```python
from build123d import *

# Parameters (mm, degrees)
F3_DEPTH = 24.4
F4_DEPTH = 2.4
F5_DEPTH = 13.4
F6_R     = 2


with BuildPart() as f3:
    # F2 (on Top) → F3 (new body)
    with BuildSketch(Plane.XY):
        with BuildLine():
            Line((-15.865, -9.0505248467), (-15.865, 0))
            Line((-15.865, 0), (-15.865, 9.0505248467))
            ThreePointArc((-15.865, 9.0505248467), (-17.6548074189, 4.68166637), (-18.265, 0))
            ThreePointArc((-18.265, 0), (-17.6548074189, -4.68166637), (-15.865, -9.0505248467))
        make_face()
        with BuildLine():
            ThreePointArc((-18.265, 0), (-17.6548074189, 4.68166637), (-15.865, 9.0505248467))
            Line((-15.865, 9.0505248467), (-15.865, 18.265))
            Line((-15.865, 18.265), (-18.265, 18.265))
            Line((-18.265, 18.265), (-18.265, 0))
        make_face()
        with BuildLine():
            Line((-15.865, -18.265), (-15.865, -9.0505248467))
            ThreePointArc((-15.865, -9.0505248467), (-17.6548074189, -4.68166637), (-18.265, 0))
            Line((-18.265, 0), (-18.265, -18.265))
            Line((-18.265, -18.265), (-15.865, -18.265))
        make_face()
        with BuildLine():
            Line((-15.865, 9.0505248467), (-15.865, 0))
            Line((-15.865, 0), (-15.865, -9.0505248467))
            ThreePointArc((-15.865, -9.0505248467), (4.68166637, -17.6548074189), (18.265, 0))
            ThreePointArc((18.265, 0), (4.68166637, 17.6548074189), (-15.865, 9.0505248467))
        make_face()
        with BuildLine():
            ThreePointArc((-15.865, 0), (0, 15.865), (15.865, 0))
            ThreePointArc((15.865, 0), (0, -15.865), (-15.865, 0))
        make_face(mode=Mode.SUBTRACT)
    extrude(amount=F3_DEPTH)

    # F2 (on Top) → F4 (join)
    with BuildSketch(Plane.XY):
        with BuildLine():
            Line((-15.865, 9.0505248467), (-15.865, 0))
            Line((-15.865, 0), (-15.865, -9.0505248467))
            ThreePointArc((-15.865, -9.0505248467), (4.68166637, -17.6548074189), (18.265, 0))
            ThreePointArc((18.265, 0), (4.68166637, 17.6548074189), (-15.865, 9.0505248467))
        make_face()
        with BuildLine():
            ThreePointArc((-15.865, 0), (0, 15.865), (15.865, 0))
            ThreePointArc((15.865, 0), (0, -15.865), (-15.865, 0))
        make_face(mode=Mode.SUBTRACT)
        with BuildLine():
            ThreePointArc((-15.865, 0), (0, -15.865), (15.865, 0))
            ThreePointArc((15.865, 0), (0, 15.865), (-15.865, 0))
        make_face()
        Polygon((-7.6111814104, 9.7325870595), (4.6230769329, 11.457769984), (12.2342583433, 1.7251829245), (7.6111814104, -9.7325870595), (-4.6230769329, -11.457769984), (-12.2342583433, -1.7251829245), align=None, mode=Mode.SUBTRACT)
        Polygon((12.2342583433, 1.7251829245), (4.6230769329, 11.457769984), (-7.6111814104, 9.7325870595), (-12.2342583433, -1.7251829245), (-4.6230769329, -11.457769984), (7.6111814104, -9.7325870595), align=None)
    extrude(amount=F4_DEPTH)

    # F2 (on Top) → F5 (join)
    with BuildSketch(Plane.XY):
        with BuildLine():
            ThreePointArc((-15.865, 0), (0, -15.865), (15.865, 0))
            ThreePointArc((15.865, 0), (0, 15.865), (-15.865, 0))
        make_face()
        Polygon((-7.6111814104, 9.7325870595), (4.6230769329, 11.457769984), (12.2342583433, 1.7251829245), (7.6111814104, -9.7325870595), (-4.6230769329, -11.457769984), (-12.2342583433, -1.7251829245), align=None, mode=Mode.SUBTRACT)
    extrude(amount=F5_DEPTH)

    # F6
    f6_edges = [f3.edges().sort_by_distance(p)[0] for p in [
        (-15.865, -9.050525, 12.2),
        (-15.865, 9.050525, 12.2),
    ]]
    fillet(f6_edges, radius=F6_R)


solid = f3.part
```
Input: part model. Units: mm. Frame: model coordinates. A direction names the side the tool comes from. Round coordinates to 2 decimals unless told otherwise and drop trailing zeros. Write each loop counter-clockwise with the first axis right and the second up, starting at its lowest first coordinate (ties: lowest second). Pieces come first, ordered by that corner, then holes. Notation, with made-up numbers: M 47,24 L 105,24 A20 ccw 105,48 Z; hole C 53,41 d3. An arc over 180 degrees is marked long. Write each question's results on one line, items separated by ' | '.
Q1. Section query B-B (x = 8.5). Return loops of the section in (y, z), and give its area (3 significant figures).
Results:
outline: M -16.17,0 L 16.17,0 L 16.17,24.4 L 13.4,24.4 L 13.4,13.4 L 6.5,13.4 L 6.5,2.4 L -7.53,2.4 L -7.53,13.4 L -13.4,13.4 L -13.4,24.4 L -16.17,24.4 Z | area: 340 mm^2
Q2. Section query D-D (z = 20). Return loops of the section in (x, y) (3 decimals).
Results:
outline: M -18.265,-18.265 L -15.865,-18.265 L -15.865,-14.779 A2 cw -12.497,-13.321 A18.265 ccw long -12.497,13.321 A2 cw -15.865,14.779 L -15.865,18.265 L -18.265,18.265 Z; hole C 0,0 d31.73
Q3. Pin query (flat end, axial travel): P1, Ø5, axis at x = 5.5, y = -11.5, coming from the -Z side; P2, Ø1.5, axis at x = -1, z = 18, coming from the -Y side; P3, Ø5, axis at y = 6, z = 17.5, coming from the +X side; P4, Ø3, axis at y = -4, z = 7, coming from the +X side. Return the tip coordinate at first contact, or that it passes through.
Results:
P1: stops at z = 0 | P2: stops at y = -18.26 | P3: stops at x = 17.93 | P4: stops at x = 18.09
Q4. Section query A-A (z = 7). Return loops of the section in (x, y) (3 decimals), and give its area (3 significant figures).
Results:
outline: M -18.265,-18.265 L -15.865,-18.265 L -15.865,-14.779 A2 cw -12.497,-13.321 A18.265 ccw long -12.497,13.321 A2 cw -15.865,14.779 L -15.865,18.265 L -18.265,18.265 Z; hole M -12.234,-1.725 L -4.623,-11.458 L 7.611,-9.733 L 12.234,1.725 L 4.623,11.458 L -7.611,9.733 Z | area: 721 mm^2
Q5. Draft query along X for faces 1 (the face through (8.375, 6.66, 7.823)), 2 (the face through (-17, 18.265, 12)), 3 (the face through (-18.265, 0, 12)). Return one class per face: released by +X, released by -X, zero draft, split by the parting line, or undercut.
Results:
face 1: undercut | face 2: zero draft | face 3: released by -X
Q6. Section query C-C (y = 6.5). Return loops of the section in (x, z) (1 decimal), and give its area (3 significant figures).
Results:
outline: M -18.3,0 L 17.1,0 L 17.1,24.4 L 14.5,24.4 L 14.5,13.4 L 8.5,13.4 L 8.5,2.4 L -8.9,2.4 L -8.9,13.4 L -14.5,13.4 L -14.5,24.4 L -18.3,24.4 Z | area: 352 mm^2
Q7. Access query for faces 4 (the face through (0, 0, 0)), 5 (the face through (-15.865, 16, 12)), 6 (the face through (-1.58, 10.583, 7.823)), 7 (the face through (-15.865, -17, 12)). Directions: +Z, -Z, +X, -X, +Y, -Y. A direction counts if a zero-diameter tool reaches every point of the face in a straight line with its end or side. Return the directions, or none.
Results:
face 4: -Z, +X, -X, +Y, -Y | face 5: +Z, -Z, +Y | face 6: +Z | face 7: +Z, -Z, -Y
Q8. Line query: line 1 along X through (y, z) = (0, 16.5) (3 decimals); line 2 along X through (y, z) = (-13.5, 21) (3 decimals). Output: solid intervals per line, ascending.
Results:
line 1: x = -18.265 to -15.865, 15.865 to 18.265 | line 2: x = -18.265 to -15.402, -12.303 to -8.334, 8.334 to 12.303
